from build123d import *

# Parameters (mm, degrees)
F0_W          = 32.5
F0_H          = 12
F1_DEPTH      = 2.4
F2_W          = 22.6
F2_H          = 12
F3_DEPTH      = 3
F3_DEPTH_BACK = 12
F4_R          = 5
F5_DEPTH      = 3
F6_R          = 2
F7_DEPTH      = 2.6


with BuildPart() as f1:
    # F0 (on Top) → F1 (new body)
    with BuildSketch(Plane.XY):
        with Locations((5.3, 0)):
            Rectangle(F0_W, F0_H)
    extrude(amount=F1_DEPTH)

    # F2 (on face) → F3 (join, two sides)
    with BuildSketch(Plane.XY.offset(2.4)) as f3_sk:
        with Locations((5.3, 0)):
            Rectangle(F2_W, F2_H)
    extrude(amount=F3_DEPTH)
    extrude(f3_sk.sketch, amount=-F3_DEPTH_BACK)

    # F4 (on face) → F5 (join)
    with BuildSketch(Plane.XY.offset(5.4)):
        Circle(F4_R)
    extrude(amount=F5_DEPTH)

    # F6 (on face) → F7 (join)
    with BuildSketch(Plane.XY.offset(8.4)):
        Circle(F6_R)
    extrude(amount=F7_DEPTH)


solid = f1.part
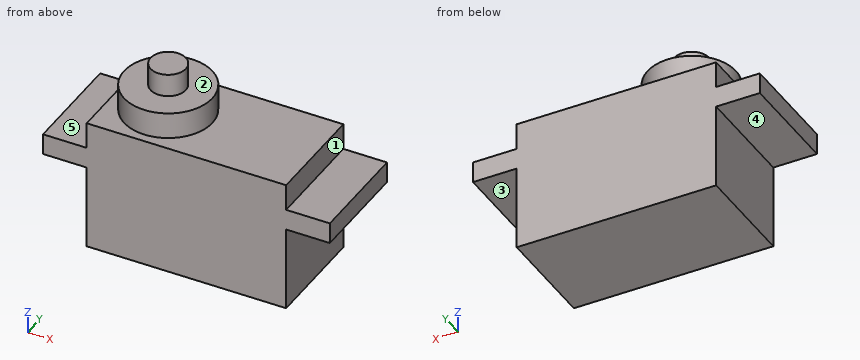
Here's how the part is built. I have some questions about the finished solid (model axes, mm). Face numbers are marked on the shaded views. A direction names the side the tool comes from. Round coordinates to 2 decimals unless told otherwise and drop trailing zeros. Order: outer loops, then holes, each group sorted by start corner. A loop starts at its lowest first (then second) coordinate and runs counter-clockwise, first axis right, second up. Notation, with made-up numbers: M 54,-26 L 75,-26 A21 ccw 75,-7 Z; hole C 89.25,-25 d5. An arc over 180 degrees is marked long. Return JSON: item names as keys, results as strings. Group by question number.
1. If we section it at A-A on y = 0: List the corners of the cut face in (x, z) for me.
2. On a 3-axis mill with a long thin cutter (end or side, diameter ignored), from which of +Z, -Z, +X, -X, +Y, -Y can I reach the whole of each face in a straight line? I mean the marked faces 1, 2, 3, 4 and 5. Say none if no direction works.
3. If we section it at B-B on x = 4: List the corners of the cut face in (y, z) for me, then the cut area to 3 significant figures.
4. Please list where these lines run through material, in increasing order: probe 1 along Z at (x, y) = (6.5, 1.75); probe 2 along X at (y, z) = (-3, -6.25); probe 3 along Z at (x, y) = (-3, -3.75).
5. I'm going to push flat-ended pins straight in: pin 1 Ø3.5 at (y, z) = (-0.5, 4) entering from +X; pin 2 Ø2.5 at (x, y) = (-9, 2.5) entering from -Z; pin 3 Ø3 at (y, z) = (1.5, -5) entering from +X; pin 4 Ø4 at (x, y) = (18.5, 1.5) entering from +Z. Where does each tip first touch, or does it pass through?
6. If we section it at C-C on z = 6.25: List the corners of the cut face in (x, y) for me, then the cut area to 3 significant figures.
7. If we section it at D-D on y = -3.25: List the corners of the cut face in (x, z) for me, then the cut area to 3 significant figures.
Reply:
{
 "1": {"outline": "M -10.95,0 L -6,0 L -6,-9.6 L 16.6,-9.6 L 16.6,0 L 21.55,0 L 21.55,2.4 L 16.6,2.4 L 16.6,5.4 L 5,5.4 L 5,8.4 L 2,8.4 L 2,11 L -2,11 L -2,8.4 L -5,8.4 L -5,5.4 L -6,5.4 L -6,2.4 L -10.95,2.4 Z"},
 "2": {"face 1": "+Z, +X, +Y, -Y", "face 2": "+Z", "face 3": "-Z, +X, +Y, -Y", "face 4": "-Z, -X, +Y, -Y", "face 5": "+Z, -X, +Y, -Y"},
 "3": {"outline": "M -6,-9.6 L 6,-9.6 L 6,5.4 L 3,5.4 L 3,8.4 L -3,8.4 L -3,5.4 L -6,5.4 Z", "area": "198 mm^2"},
 "4": {"probe 1": "-9.6 to 5.4", "probe 2": "-6 to 16.6", "probe 3": "-9.6 to 8.4"},
 "5": {"pin 1": "x = 21.55", "pin 2": "z = 0", "pin 3": "x = 16.6", "pin 4": "z = 5.4"},
 "6": {"outline": "C 0,0 d10", "area": "78.5 mm^2"},
 "7": {"outline": "M -10.95,0 L -6,0 L -6,-9.6 L 16.6,-9.6 L 16.6,0 L 21.55,0 L 21.55,2.4 L 16.6,2.4 L 16.6,5.4 L 3.8,5.4 L 3.8,8.4 L -3.8,8.4 L -3.8,5.4 L -6,5.4 L -6,2.4 L -10.95,2.4 Z", "area": "386 mm^2"}
}
